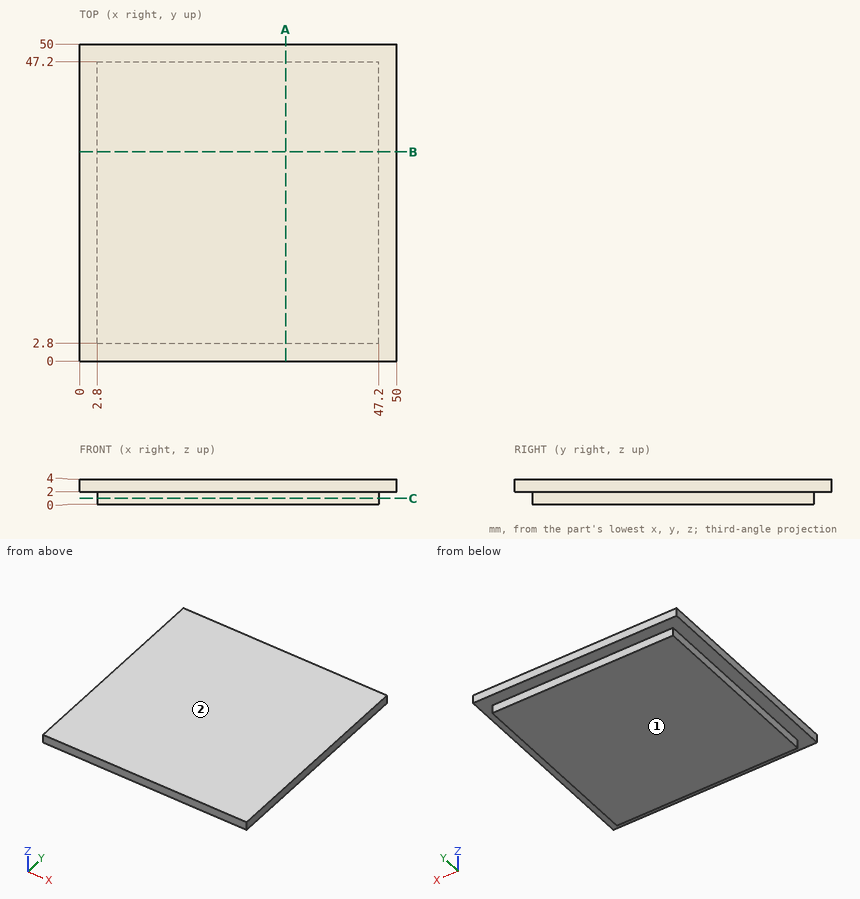
Design review of the part shown in the three views and the two pictorial views. Dimensions are in mm from the part's minimum x, y and z. Coordinates: 2 decimals unless noted, no trailing zeros. Write each loop counter-clockwise with the first axis right and the second up, starting at its lowest first coordinate (ties: lowest second). Pieces come first, ordered by that corner, then holes.
1) We need section A-A on x = 32.5. State the section outline as (y, z) points, then the cut area to 3 significant figures.
2) The part is to be moulded in two halves that separate along Z. For the marked faces 1 and 2, say which applies: pulls with the +Z half, pulls with the -Z half, needs draft (parallel to the pull), parting line crosses it, or undercut.
3) To check wall thickness, follow probe 1 along Y at (x, z) = (47, 1.95); probe 2 along Z at (x, y) = (48, 33). State the ranges of each line that lie inside material, in increasing order.
4) We need section C-C on z = 0.95. State the section outline as (x, y) points, then the cut area to 3 significant figures.
5) Clearance check with flat-ended pins moving along their axes: pin 1 Ø2 at (y, z) = (23, 1.5) entering from -X; pin 2 Ø1 at (x, z) = (32.5, 1) entering from +Y; pin 3 Ø0.6 at (y, z) = (29.5, 1.5) entering from +X; pin 4 Ø1 at (x, z) = (31.5, 0.5) entering from -Y. State where each tip first meets the part, or that it passes through.
Answer list:
1. outline: (0, 2) - (2.8, 2) - (2.8, 0) - (47.2, 0) - (47.2, 2) - (50, 2) - (50, 4) - (0, 4) - close
1. area: 189 mm2
2. face 1: pulls with the -Z half
2. face 2: pulls with the +Z half
3. probe 1: y = 2.8 to 47.2
3. probe 2: z = 2 to 4
4. outline: (2.8, 2.8) - (47.2, 2.8) - (47.2, 47.2) - (2.8, 47.2) - close
4. area: 1,970 mm2
5. pin 1: stops at x = 0
5. pin 2: stops at y = 47.2
5. pin 3: stops at x = 47.2
5. pin 4: stops at y = 2.8
